Model file for the job. Use its own axes, mm. A direction names the side the tool comes from. Give positions to 0.01 mm unless a question says otherwise; leave off trailing zeros. Loops run counter-clockwise (first coordinate to the right, second up) from the corner with the lowest first, then second, coordinate; pieces in that order, holes last. Notation, with made-up numbers: (-20, 11) -> (-15, 11) arc R23 ccw to (-15, 46) -> close; hole circle Ø4 at (53.5, -7.5). An arc over 180 degrees is marked (long way). Use CSV: the item, a comma, the result in double quotes. Start each with the question number.
(1) Cut at C-C on z = 1.55. State how many separate pieces and enclosed holes the cut face has, then the cut area to 3 significant figures.
(2) Flat gauge pin, fed straight in: pin 1 (4 mm diameter, centred on x = 69.85, y = -203.2, fed in from -Z). Where does the tip first touch, or does it go through?
(3) Cut at B-B on y = -127. Write the cut outline in (x, z) (3 decimals), then the cut area to 3 significant figures.
(4) Drill centre lines: probe 1 along Y at (x, z) = (127, 1.45); probe 2 along X at (y, z) = (-209.55, 1) (3 decimals); probe 3 along Y at (x, z) = (-69.85, 1.7). Where is each one in solid material? Low to high.
(5) Pull direction Y, two halves, no side cores. Call faces 3 (the cylindrical face through (160.637, -204.038, 1.565)), 4 (the flat face through (42, -189, 3.175)), 5 (the cylindrical face through (-175.89, -226.79, 1.57)): pulls with the +Y half, pulls with the -Y half, needs draft (parallel to the pull), parting line crosses it, or undercut.
(6) Cut at D-D on x = -106. Write the cut outline in (y, z) (3 decimals).
(7) 3-axis set-ups, long thin cutter, end or side, ignore diameter. For faces 1 (the cylindrical face through (-113.41, -170.16, 1.57)), 2 (the cylindrical face through (131.075, -15.744, 1.565)): which of +Z, -Z, +X, -X, +Y, -Y reach the whole face in a straight line?
(8) Cut at A-A on x = 19.05. Write the cut outline in (y, z) (3 decimals), then the cut area to 3 significant figures.
from build123d import *

# Parameters (mm, degrees)
SKETCH1_R           = 14.2875
SKETCH1_R_2         = 19.05
SKETCH1_R_3         = 2.54
SKETCH1_R_4         = 5.715
BOSS_EXTRUDE3_DEPTH = 3.175
SKETCH2_W           = 355.6
SKETCH2_H           = 19.05
CUT_EXTRUDE1_DEPTH  = 290.621961572
FILLET1_R           = 19.05


with BuildPart() as part:
    # Sketch1 → Boss-Extrude3 (new body)
    with BuildSketch(Plane.XY):
        with BuildLine():
            Line((120.65, -152.4), (120.65, -6.35))
            Line((120.65, -6.35), (120.65, 6.35))
            ThreePointArc((120.65, 6.35), (124.369743879, 15.330256121), (133.35, 19.05))
            Line((133.35, 19.05), (165.1, 19.05))
            ThreePointArc((165.1, 19.05), (174.080256121, 15.330256121), (177.8, 6.35))
            Line((177.8, 6.35), (177.8, -6.35))
            Line((177.8, -6.35), (177.8, -222.25))
            ThreePointArc((177.8, -222.25), (175.940128061, -226.740128061), (171.45, -228.6))
            Line((171.45, -228.6), (12.7, -228.6))
            Line((12.7, -228.6), (-12.7, -228.6))
            Line((-12.7, -228.6), (-171.45, -228.6))
            ThreePointArc((-171.45, -228.6), (-175.940128061, -226.740128061), (-177.8, -222.25))
            Line((-177.8, -222.25), (-177.8, -6.35))
            Line((-177.8, -6.35), (-177.8, 6.35))
            ThreePointArc((-177.8, 6.35), (-174.080256121, 15.330256121), (-165.1, 19.05))
            Line((-165.1, 19.05), (-133.35, 19.05))
            ThreePointArc((-133.35, 19.05), (-124.369743879, 15.330256121), (-120.65, 6.35))
            Line((-120.65, 6.35), (-120.65, -6.35))
            Line((-120.65, -6.35), (-120.65, -152.4))
            ThreePointArc((-120.65, -152.4), (-113.210512242, -170.360512242), (-95.25, -177.8))
            Line((-95.25, -177.8), (-12.7, -177.8))
            Line((-12.7, -177.8), (12.7, -177.8))
            Line((12.7, -177.8), (95.25, -177.8))
            ThreePointArc((95.25, -177.8), (113.210512242, -170.360512242), (120.65, -152.4))
        make_face()
        with Locations((141.605, -25.4)):
            Circle(SKETCH1_R, mode=Mode.SUBTRACT)
        with Locations(Location((-141.605, -25.4, 0), (0, 0, 180))):
            Circle(SKETCH1_R, mode=Mode.SUBTRACT)
        with Locations((-141.605, -203.2)):
            Circle(SKETCH1_R_2, mode=Mode.SUBTRACT)
        with Locations(Location((141.605, -203.2, 0), (0, 0, 180))):
            Circle(SKETCH1_R_2, mode=Mode.SUBTRACT)
        with Locations((-69.85, -203.2)):
            Circle(SKETCH1_R_3, mode=Mode.SUBTRACT)
        with Locations(Location((69.85, -203.2, 0), (0, 0, 180))):
            Circle(SKETCH1_R_3, mode=Mode.SUBTRACT)
        with Locations((-19.05, -203.2)):
            Circle(SKETCH1_R_4, mode=Mode.SUBTRACT)
        with Locations((-149.225, 6.35)):
            Circle(SKETCH1_R_3, mode=Mode.SUBTRACT)
        with Locations(Location((149.225, 6.35, 0), (0, 0, 180))):
            Circle(SKETCH1_R_3, mode=Mode.SUBTRACT)
        with Locations((-168.275, -209.55)):
            Circle(SKETCH1_R_3, mode=Mode.SUBTRACT)
        with Locations(Location((168.275, -209.55, 0), (0, 0, 180))):
            Circle(SKETCH1_R_3, mode=Mode.SUBTRACT)
        with Locations((-165.1, -76.2)):
            Circle(SKETCH1_R_3, mode=Mode.SUBTRACT)
        with Locations(Location((165.1, -76.2, 0), (0, 0, 180))):
            Circle(SKETCH1_R_3, mode=Mode.SUBTRACT)
        with Locations((-127, -171.45)):
            Circle(SKETCH1_R_3, mode=Mode.SUBTRACT)
        with Locations(Location((127, -171.45, 0), (0, 0, 180))):
            Circle(SKETCH1_R_3, mode=Mode.SUBTRACT)
        with Locations(Location((19.05, -203.2, 0), (0, 0, 180))):
            Circle(SKETCH1_R_4, mode=Mode.SUBTRACT)
    extrude(amount=BOSS_EXTRUDE3_DEPTH)

    # Sketch2 → Cut-Extrude1 (cut, through all)
    with BuildSketch(Plane.XY.offset(3.175)):
        with Locations((0, 9.525)):
            Rectangle(SKETCH2_W, SKETCH2_H)
    extrude(amount=-CUT_EXTRUDE1_DEPTH, mode=Mode.SUBTRACT)

    # Fillet1
    fillet1_edges = [part.edges().sort_by_distance(p)[0] for p in [
        (-177.8, 0, 1.5875),
        (120.65, 0, 1.5875),
        (177.8, 0, 1.5875),
        (-120.65, 0, 1.5875),
    ]]
    fillet(fillet1_edges, radius=FILLET1_R)


solid = part.part
Check result:
1,separate pieces,"1"
1,enclosed holes,"14"
1,area,"34,400 mm²"
2,pin 1,"through"
3,outline,"(-177.8, 0) -> (-120.65, 0) -> (-120.65, 3.175) -> (-177.8, 3.175) -> close; (120.65, 0) -> (177.8, 0) -> (177.8, 3.175) -> (120.65, 3.175) -> close"
3,area,"363 mm²"
4,probe 1,"-228.6 to -215.43, -190.97 to -173.99, -168.91 to -4.85"
4,probe 2,"-177.8 to -170.815, -165.735 to -159.566, -123.644 to 123.644, 159.566 to 165.735, 170.815 to 177.8"
4,probe 3,"-228.6 to -205.74, -200.66 to -177.8"
5,face 3,"undercut"
5,face 4,"needs draft"
5,face 5,"pulls with the -Y half"
6,outline,"(-228.6, 0) -> (-175.413, 0) -> (-175.413, 3.175) -> (-228.6, 3.175) -> close"
7,face 1,"+Z, -Z, +Y"
7,face 2,"+Z, -Z"
8,outline,"(-228.6, 0) -> (-208.915, 0) -> (-208.915, 3.175) -> (-228.6, 3.175) -> close; (-197.485, 0) -> (-177.8, 0) -> (-177.8, 3.175) -> (-197.485, 3.175) -> close"
8,area,"125 mm²"
